Read the model definition and answer for the solid it produces. Units are mm, in the model's axes. Face numbers are marked on the shaded views. A direction names the side the tool comes from. Coordinates: 2 decimals unless noted, no trailing zeros. Write each loop counter-clockwise with the first axis right and the second up, starting at its lowest first coordinate (ties: lowest second). Pieces come first, ordered by that corner, then holes. Notation, with made-up numbers: (4.5, 59) -> (29.5, 59) arc R28 cw to (29.5, 98) -> close; hole circle Ø9 at (-10, 68.25). An arc over 180 degrees is marked (long way). Answer in a Markdown table with one row per item. Add a question column.
Item 1: For a pull along Z with two mould halves and no side action, classify the marked faces 3, 4, 5 and 6 as +Z half, -Z half, draft (parallel to the pull), parting line (faces both ways), or undercut.
Item 2: Which of the six approach directions +Z, -Z, +X, -X, +Y, -Y give full straight-line access (tool end or side, diameter ignored) to the marked faces 1 and 2?
Item 3: Given pin 1 Ø1 at (y, z) = (7.5, -1.5) entering from -X; pin 2 Ø0.5 at (y, z) = (-15, -0.5) entering from +X; pin 3 Ø3.5 at (x, z) = (29, 16) entering from +Y; pin 4 Ø3 at (x, z) = (27.5, -0.5) entering from -Y, each flat-ended and moving along its own axis, determine where each tip first touches the part or whether it passes through.
Item 4: Section B-B on y = -2 is taken. Write down the section's boundary in (x, z).
Item 5: Straight lines are drawn through the part: line 1 (Z direction, x = 29, y = 11.75); line 2 (X direction, y = 8, z = -16); line 3 (Z direction, x = 24.5, y = 0). For each, find the intervals that lie inside material, in ascending order. Write a range as from..to.
Item 6: Section A-A on y = 9.5 is taken. Write down the section's boundary in (x, z), then the cut area to 3 significant figures.
Autodesk Inventor part; units mm, degrees
ref_plane "bnt_nut_1_XY" through (0, 0, 0) normal (1, 0, 0) x (0, 0, -1)
ref_plane "bnt_nut_1_YZ" through (0, 0, 0) normal (0, 0, -1) x (0, 1, 0)
ref_plane "bnt_nut_1_ZX" through (0, 0, 0) normal (0, 1, 0) x (1, 0, 0)
sketch "Sketch_1" plane through (0, 0, 0) normal (1, 0, 0) x (0, 1, 0)
  line L0 (14.74, 21) -> (-5.5, 21)
  line L1 (-5.5, 21) -> (-6.76, 19.74)
  line L2 (-6.76, 19.74) -> (-9.76, 19.74)
  line L3 (-9.76, 19.74) -> (-9.76, 15.75)
  arc A0 (-9.76, 15.75) -> (-13.25, 8.26) centre (1.867, 5.7743) ccw
  line L4 (-13.25, 8.26) -> (-13.25, -8.26)
  arc A1 (-13.25, -8.26) -> (-9.76, -15.75) centre (1.867, -5.7743) ccw
  line L5 (-9.76, -15.75) -> (-9.76, -19.74)
  line L6 (-9.76, -19.74) -> (-6.76, -19.74)
  line L7 (-6.76, -19.74) -> (-5.5, -21)
  line L8 (-5.5, -21) -> (14.74, -21)
  line L9 (14.74, -21) -> (16, -19.74)
  line L10 (16, -19.74) -> (16, -8.26)
  line L11 (16, -8.26) -> (14.74, -7)
  line L12 (14.74, -7) -> (14.74, 7)
  line L13 (14.74, 7) -> (16, 8.26)
  line L14 (16, 8.26) -> (16, 19.74)
  line L15 (16, 19.74) -> (14.74, 21)
  circle A2 centre (0, 0) radius 8
extrude "Extrusion1" add sketch "Sketch_1" along normal blind 36
sketch "Sketch_2" plane through (18, 0, 0) normal (0.682, 0, 0.7314) x (0.7314, 0, -0.682)
  line L0 (-18, -14.0625) -> (-3.1468, -14.0625)
  arc A0 (-3.1468, -14.0625) -> (3.1468, -14.0625) centre (0, -13.25) ccw
  line L1 (3.1468, -14.0625) -> (18, -14.0625)
  line L2 (18, -14.0625) -> (18, -13.25)
  line L3 (18, -13.25) -> (-18, -13.25)
  line L4 (-18, -13.25) -> (-18, -14.0625)
extrude "Extrusion2" add sketch "Sketch_2" along normal mid plane 36
sketch "Sketch_3" plane through (0, -13.25, 0) normal (0, 1, 0) x (1, 0, 0)
  line L0 (-18, -36) -> (54, -36)
  line L1 (54, -36) -> (54, 36)
  line L2 (54, 36) -> (-18, 36)
  line L3 (-18, 36) -> (-18, -36)
  line L4 (6, -8.26) -> (30, -8.26)
  line L5 (30, -8.26) -> (30, 8.26)
  line L6 (30, 8.26) -> (6, 8.26)
  line L7 (6, 8.26) -> (6, -8.26)
extrude "Extrusion3" cut sketch "Sketch_3" against normal blind 3.25
sketch "Sketch_4" plane through (0, 0, 0) normal (0, 0, 1) x (1, 0, 0)
  line L0 (8.34, -15.3425) -> (8.34, -14.0625)
  line L1 (8.34, -14.0625) -> (9.94, -14.0625)
  line L2 (9.94, -14.0625) -> (9.94, -15.0225)
  arc A0 (9.62, -15.3425) -> (9.94, -15.0225) centre (9.62, -15.0225) ccw
  line L3 (9.62, -15.3425) -> (8.34, -15.3425)
  line L4 (8.34, -15.3425) -> (8.34, -14.0625)
revolve "Revolution1" add sketch "Sketch_4" angle 360 about axis through (8.34, -15.3425, 0) along (0, -1, 0)
sketch "Sketch_5" plane through (0, 0, 0) normal (0, 0, 1) x (1, 0, 0)
  line L0 (27.66, -15.3425) -> (27.66, -14.0625)
  line L1 (27.66, -14.0625) -> (29.26, -14.0625)
  line L2 (29.26, -14.0625) -> (29.26, -15.0225)
  arc A0 (28.94, -15.3425) -> (29.26, -15.0225) centre (28.94, -15.0225) ccw
  line L3 (28.94, -15.3425) -> (27.66, -15.3425)
  line L4 (27.66, -15.3425) -> (27.66, -14.0625)
revolve "Revolution2" add sketch "Sketch_5" angle 360 about axis through (27.66, -15.3425, 0) along (0, -1, 0)
sketch "Sketch_6" plane through (0, -15.3425, 0) normal (0, 1, 0) x (1, 0, 0)
  line L0 (26.86, 0.15) -> (26.86, -0.15)
  line L1 (26.86, -0.15) -> (27.51, -0.15)
  line L2 (27.51, -0.15) -> (27.51, -0.8)
  line L3 (27.51, -0.8) -> (27.81, -0.8)
  line L4 (27.81, -0.8) -> (27.81, -0.15)
  line L5 (27.81, -0.15) -> (28.46, -0.15)
  line L6 (28.46, -0.15) -> (28.46, 0.15)
  line L7 (28.46, 0.15) -> (27.81, 0.15)
  line L8 (27.81, 0.15) -> (27.81, 0.8)
  line L9 (27.81, 0.8) -> (27.51, 0.8)
  line L10 (27.51, 0.8) -> (27.51, 0.15)
  line L11 (27.51, 0.15) -> (26.86, 0.15)
extrude "Extrusion4" cut sketch "Sketch_6" along normal blind 0.64
sketch "Sketch_7" plane through (0, -15.3425, 0) normal (0, 1, 0) x (1, 0, 0)
  line L0 (7.54, 0.15) -> (7.54, -0.15)
  line L1 (7.54, -0.15) -> (8.19, -0.15)
  line L2 (8.19, -0.15) -> (8.19, -0.8)
  line L3 (8.19, -0.8) -> (8.49, -0.8)
  line L4 (8.49, -0.8) -> (8.49, -0.15)
  line L5 (8.49, -0.15) -> (9.14, -0.15)
  line L6 (9.14, -0.15) -> (9.14, 0.15)
  line L7 (9.14, 0.15) -> (8.49, 0.15)
  line L8 (8.49, 0.15) -> (8.49, 0.8)
  line L9 (8.49, 0.8) -> (8.19, 0.8)
  line L10 (8.19, 0.8) -> (8.19, 0.15)
  line L11 (8.19, 0.15) -> (7.54, 0.15)
extrude "Extrusion5" cut sketch "Sketch_7" along normal blind 0.64
sketch "Sketch8" plane through (0, -5.5, 21) normal (0, 0, 1) x (1, 0, 0)
  point P0 (6, 3.5)
hole "Hole1" at (6, -2, 21) direction (0, 0, -1) diameter 4.917 depth 13.5806 tip angle 120 countersink diameter 6 countersink angle 90
sketch "Sketch9" plane through (0, 16, -8.26) normal (0, 1, 0) x (1, 0, 0)
  point P0 (7, 7.74)
hole "Hole2" at (7, 16, -16) direction (0, -1, 0) diameter 4.134 depth 10.5066 tip angle 120 countersink diameter 5 countersink angle 90
pattern_linear "Rectangular Pattern1" count 2 spacing 22 along (1, 0, 0) count 2 spacing 32 along (0, 0, 1) of "Hole2"
ref_plane "bnt_nut_1_XY" through (0, 0, 0) normal (1, 0, 0) x (0, 0, -1)
ref_plane "bnt_nut_1_YZ" through (0, 0, 0) normal (0, 0, -1) x (0, 1, 0)
ref_plane "bnt_nut_1_ZX" through (0, 0, 0) normal (0, 1, 0) x (1, 0, 0)
thread "Thread1"
properties part number "BNT 1605-2.6 Nut"
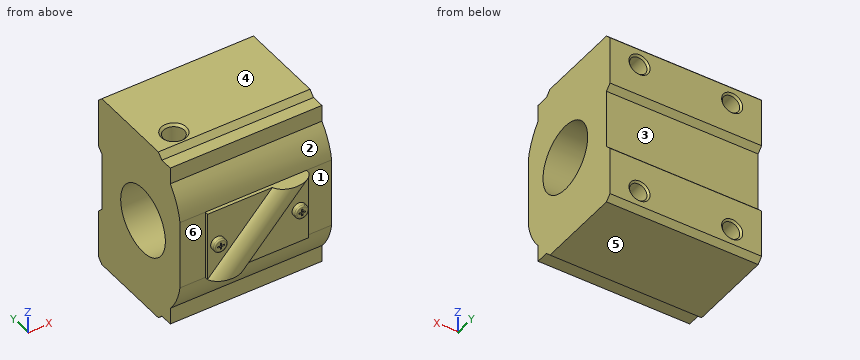
Results below:
| question | item | result |
|---|---|---|
| 1 | face 3 | undercut |
| 1 | face 4 | +Z half |
| 1 | face 5 | -Z half |
| 1 | face 6 | draft |
| 2 | face 1 | +Z, -Z, +X, -Y |
| 2 | face 2 | +Z, +X, -X, -Y |
| 3 | pin 1 | stops at x = 0 |
| 3 | pin 2 | stops at x = 29.24 |
| 3 | pin 3 | stops at y = 5.31 |
| 3 | pin 4 | stops at y = -15.34 |
| 4 | outline | (0, -21) -> (36, -21) -> (36, -7.75) -> (0, -7.75) -> close; (0, 7.75) -> (3.54, 7.75) -> (3.54, 20.46) -> (3, 21) -> (0, 21) -> close; (8.46, 7.75) -> (36, 7.75) -> (36, 21) -> (9, 21) -> (8.46, 20.46) -> close |
| 5 | line 1 | z = -21..-18.07, -13.93..13.93, 18.07..21 |
| 5 | line 2 | x = 0..4.93, 9.07..26.93, 31.07..36 |
| 5 | line 3 | z = -21..-8, 8..21 |
| 6 | outline | (0, -21) -> (36, -21) -> (36, 21) -> (0, 21) -> close; hole circle Ø4.13 at (7, -16); hole circle Ø4.13 at (7, 16); hole circle Ø4.13 at (29, -16); hole circle Ø4.13 at (29, 16) |
| 6 | area | 1,460 mm2 |
